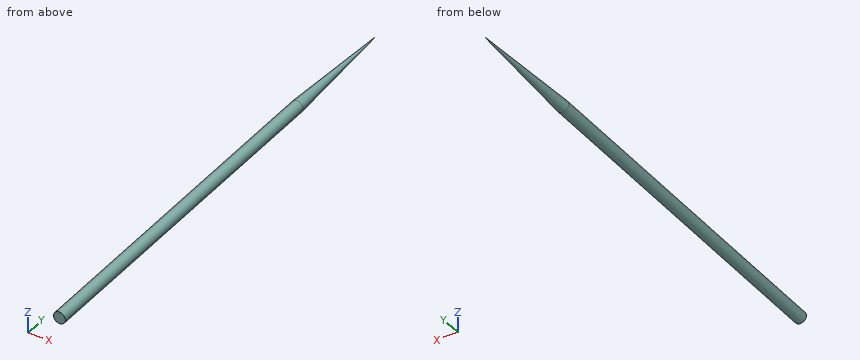
```python
from build123d import *

# Parameters (mm, degrees)
SKETCH_1_R    = 0.5
SCALE_1_SCALE = 0.7


with BuildPart() as part:
    # По траектории1: sweep along a path in Эскиз2
    with BuildLine(Plane.XY) as sweep_1_path:
        Line((0, -20.788855077), (0, 9.211144923))
    # Эскиз1 → По траектории1 (sweep)
    with BuildSketch(Plane(origin=(0, 0, 0), x_dir=(1, 0, 0), z_dir=(0, 1, 0))):
        Circle(SKETCH_1_R)
    sweep(path=sweep_1_path.line)

    # Эскиз5 → Повернуть1 (revolve)
    with BuildSketch(Plane(origin=(0, 0, 0), x_dir=(0, 0, -1), z_dir=(1, 0, 0)), mode=Mode.PRIVATE) as revolve_1_sk:
        Polygon((0, 19.211144923), (0.5, 9.211144923), (0, 9.211144923), align=None)
    revolve(revolve_1_sk.sketch.rotate(Axis((0, 9.211144923, 0), (0, 1, 0)), 180), axis=Axis((0, 9.211144923, 0), (0, 1, 0)))


with BuildPart() as part_1:
    # Масштаб1: scaled about (0, -4.038855077, 0)
    add(part.part.scale(SCALE_1_SCALE).moved(Location((0, -1.211656523, 0))))


solid = part_1.part
```
The model under review builds one solid part; all positions refer to its coordinate system, in mm. Give positions to 0.01 mm unless a question says otherwise; leave off trailing zeros. Write each loop counter-clockwise with the first axis right and the second up, starting at its lowest first coordinate (ties: lowest second). Pieces come first, ordered by that corner, then holes.
(1) Consider section A-A, the plane y = 3.5. Give the boundary of the cut face in (x, z), and give its area (3 significant figures).
(2) To check wall thickness, follow L1, parallel to X at y = -10.25, z = 0.05; L2, parallel to Z at x = 0.2, y = 3.75; L3, parallel to Z at x = -0.3, y = -5. State the ranges of each line that lie inside material, in increasing order.
(3) Consider section B-B, the plane y = 8.5. Give the boundary of the cut face in (x, z), and give its area (3 significant figures).
Returned:
1. outline: circle Ø0.7 at (0, 0)
1. area: 0.385 mm2
2. L1: x = -0.35 to 0.35
2. L2: z = -0.29 to 0.29
2. L3: z = -0.18 to 0.18
3. outline: circle Ø0.37 at (0, 0)
3. area: 0.110 mm2
